from build123d import *

# Parameters (mm, degrees)
F0_W     = 20
F0_H     = 30
F0_R     = 5
F1_DEPTH = 2
F2_R     = 5
F3_DEPTH = 2
F4_W     = 20
F4_H     = 2
F5_DEPTH = 2
F6_R     = 1
F7_R     = 1
F8_R     = 3


with BuildPart() as f1:
    # F0 (on Top) → F1 (new body)
    with BuildSketch(Plane.XY):
        with Locations((10, 15)):
            Rectangle(F0_W, F0_H)
        with Locations((10, 10)):
            Circle(F0_R, mode=Mode.SUBTRACT)
    extrude(amount=F1_DEPTH)

    # F2 (on face) → F3 (join)
    with BuildSketch(Plane(origin=(0, 30, 0), x_dir=(-1, 0, 0), z_dir=(0, 1, 0))):
        Polygon((-20, 7), (-20, 2), (0, 2), (0, 32), (-20, 32), (-20, 12), (-16, 12), (-16, 7), align=None)
        with Locations((-10, 22)):
            Circle(F2_R, mode=Mode.SUBTRACT)
    extrude(amount=F3_DEPTH)

    # F4 (on face) → F5 (join)
    with BuildSketch(Plane(origin=(0, 30, 0), x_dir=(-1, 0, 0), z_dir=(0, 1, 0))):
        with Locations((-10, 1)):
            Rectangle(F4_W, F4_H)
    extrude(amount=F5_DEPTH)

    # F6
    f6_edges = [f1.edges().sort_by_distance(p)[0] for p in [
        (20, 0, 1),
        (0, 0, 1),
        (20, 31, 32),
        (0, 31, 32),
    ]]
    fillet(f6_edges, radius=F6_R)

    # F7
    f7_edges = [f1.edges().sort_by_distance(p)[0] for p in [
        (10, 30, 2),
    ]]
    fillet(f7_edges, radius=F7_R)

    # F8
    f8_edges = [f1.edges().sort_by_distance(p)[0] for p in [
        (10, 32, 0),
    ]]
    fillet(f8_edges, radius=F8_R)


solid = f1.part
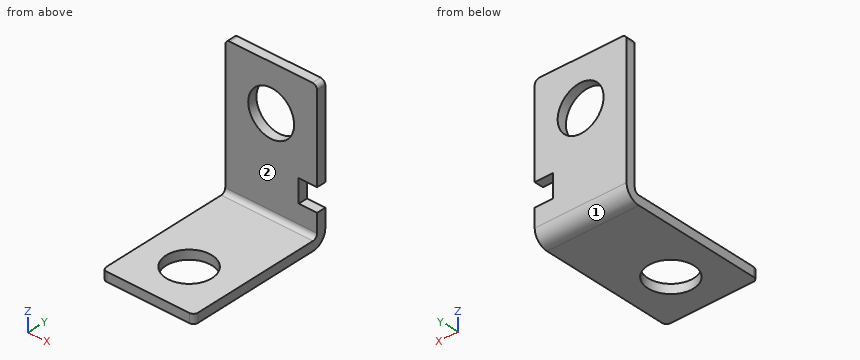
Read the model definition and answer for the solid it produces. Units are mm, in the model's axes. Face numbers are marked on the shaded views. A direction names the side the tool comes from. Coordinates: 2 decimals unless noted, no trailing zeros. Order: outer loops, then holes, each group sorted by start corner. A loop starts at its lowest first (then second) coordinate and runs counter-clockwise, first axis right, second up. Notation, with made-up numbers: (32, -20) - (53, -20) arc R21 ccw to (53, -5) - close; hole circle Ø3 at (60, -4). An arc over 180 degrees is marked (long way). Use one line per item in the form item = value.
(1) Section B-B, the plane z = 22 is taken. Give the vertices of the cut face in (x, y), then the cut area to 3 significant figures.
Computed values:
outline = (0, 30) - (5, 30) - (5, 32) - (0, 32) - close; (15, 30) - (20, 30) - (20, 32) - (15, 32) - close
area = 20.0 mm²
(2) Section A-A, the plane x = 16.75 is taken. Give the vertices of the cut face in (y, z).
Computed values:
outline = (0, 0) - (29, 0) arc R3 ccw to (32, 3) - (32, 7) - (30, 7) - (30, 3) arc R1 cw to (29, 2) - (0, 2) - close; (30, 12) - (32, 12) - (32, 32) - (30, 32) - close
(3) Given pin 1 Ø2 at (y, z) = (31, 10.5) entering from +X; pin 2 Ø1.6 at (x, y) = (18.5, 30.5) entering from -Z; pin 3 Ø4 at (x, y) = (16.5, 7.5) entering from +Z, each flat-ended and moving along its own axis, determine where each tip first touches the part or whether it passes through.
Computed values:
pin_1 = 16
pin_2 = 0.08
pin_3 = 2
(4) Section D-D, the plane x = 10 is taken. Give the vertices of the cut face in (y, z).
Computed values:
outline = (0, 0) - (5, 0) - (5, 2) - (0, 2) - close; (15, 0) - (29, 0) arc R3 ccw to (32, 3) - (32, 17) - (30, 17) - (30, 3) arc R1 cw to (29, 2) - (15, 2) - close; (30, 27) - (32, 27) - (32, 32) - (30, 32) - close
(5) Which of the six approach directions +Z, -Z, +X, -X, +Y, -Y give full straight-line access (tool end or side, diameter ignored) to the marked faces 1 and 2?
Computed values:
face_1 = -Z, +X, -X, +Y
face_2 = +Z, +X, -X, -Y
(6) Straight lines are drawn through the part: L1, parallel to Y at x = 8, z = 14.5; L2, parallel to Z at x = 8.5, y = 4.5; L3, parallel to Y at x = 10, z = 1.45. For each, find the intervals that lie inside material, in ascending order.
Computed values:
L1 = 30 to 32
L2 = 0 to 2
L3 = 0 to 5, 15 to 31.57
(7) Section C-C, the plane y = 10 is taken. Give the vertices of the cut face in (x, z).
Computed values:
outline = (0, 0) - (5, 0) - (5, 2) - (0, 2) - close; (15, 0) - (20, 0) - (20, 2) - (15, 2) - close
